from build123d import *

# Parameters (mm, degrees)
SKETCH1_R               = 6.5
BOSS_EXTRUDE1_DEPTH     = 4.64
SKETCH2_R               = 5.075
BOSS_EXTRUDE2_DEPTH     = 2
BOSS_EXTRUDE3_START     = 2
SKETCH3_R               = 5.075
BOSS_EXTRUDE3_DEPTH     = 2
SKETCH4_R               = 3.175
CUT_EXTRUDE1_DEPTH      = 13.615450844
CUT_EXTRUDE2_DEPTH      = 12.339735447
CUT_EXTRUDE2_DEPTH_BACK = 12.339735447
CUT_EXTRUDE3_DEPTH      = 12.339735447
CUT_EXTRUDE3_DEPTH_BACK = 12.339735447
SKETCH6_W               = 1
SKETCH6_H               = 2


with BuildPart() as part:
    # Sketch1 → Boss-Extrude1 (new body)
    with BuildSketch(Plane(origin=(0, 0, 0), x_dir=(1, 0, 0), z_dir=(0, 1, 0))):
        with Locations(Location((0, 0, 0), (0, 0, 270))):
            Circle(SKETCH1_R)
    extrude(amount=BOSS_EXTRUDE1_DEPTH)

    # Sketch2 → Boss-Extrude2 (add)
    with BuildSketch(Plane(origin=(0, 4.64, 0), x_dir=(1, 0, 0), z_dir=(0, 1, 0))):
        with Locations(Location((0, 0, 0), (0, 0, 270))):
            Circle(SKETCH2_R)
    extrude(amount=BOSS_EXTRUDE2_DEPTH)

    # Sketch3 → Boss-Extrude3 (add)
    with BuildSketch(Plane.XZ.offset(BOSS_EXTRUDE3_START)):
        with Locations(Location((0, 0, 0), (0, 0, 90))):
            Circle(SKETCH3_R)
    extrude(amount=-BOSS_EXTRUDE3_DEPTH)

    # Sketch4 → Cut-Extrude1 (cut, through all)
    with BuildSketch(Plane(origin=(0, 6.64, 0), x_dir=(1, 0, 0), z_dir=(0, 1, 0))):
        with Locations(Location((0, 0, 0), (0, 0, 270))):
            Circle(SKETCH4_R)
    extrude(amount=-CUT_EXTRUDE1_DEPTH, mode=Mode.SUBTRACT)

    # Sketch5 → Cut-Extrude2 (cut, two sides: drawn at the far end of the back side and taken through both)
    with BuildSketch(Plane.XY.offset(-CUT_EXTRUDE2_DEPTH_BACK)):
        Polygon((0, 0), (-1, 0), (-1, -2), (1, -2), (1, 0), align=None)
    extrude(amount=CUT_EXTRUDE2_DEPTH + CUT_EXTRUDE2_DEPTH_BACK, mode=Mode.SUBTRACT)

    # Sketch6 → Cut-Extrude3 (cut, two sides: drawn at the far end of the back side and taken through both)
    with BuildSketch(Plane(origin=(0, 0, 0), x_dir=(0, 0, -1), z_dir=(1, 0, 0)).offset(-CUT_EXTRUDE3_DEPTH_BACK)):
        with Locations((0.5, -1)):
            Rectangle(SKETCH6_W, SKETCH6_H)
        with Locations((-0.5, -1)):
            Rectangle(SKETCH6_W, SKETCH6_H)
    extrude(amount=CUT_EXTRUDE3_DEPTH + CUT_EXTRUDE3_DEPTH_BACK, mode=Mode.SUBTRACT)


solid = part.part
Input: part model. Units: mm. Frame: model coordinates. A direction names the side the tool comes from. Give positions to 0.01 mm unless a question says otherwise; leave off trailing zeros. Write each loop counter-clockwise with the first axis right and the second up, starting at its lowest first coordinate (ties: lowest second). Pieces come first, ordered by that corner, then holes.
Q1. Section C-C, the plane y = 5.25. Output: boundary loops of the cut face in (x, z) (3 decimals), plus the area to 3 significant figures.
Q2. Pull-direction query (Z, two-part tool) for faces 6 (the face through (-1, -1, 4)), 7 (the face through (3.559, -1.014, -3.618)), 8 (the face through (-4, -1, 1)); classes: pulls with the +Z half, pulls with the -Z half, needs draft (parallel to the pull), parting line crosses it, or undercut.
Q3. Material intervals for probe 1 along X at (y, z) = (4, 0) (3 decimals); probe 2 along X at (y, z) = (4.75, 0) (3 decimals); probe 3 along Y at (x, z) = (5, -2), sorted ascending.
Q4. Section D-D, the plane x = 3.75. Output: boundary loops of the cut face in (y, z).
Q5. Section A-A, the plane x = 0. Output: boundary loops of the cut face in (y, z) (3 decimals).
Q6. Section B-B, the plane z = 0. Output: boundary loops of the cut face in (x, y) (3 decimals), plus the area to 3 significant figures.
Q7. Set-up query: faces 1 (the face through (-5, 4.64, -2)), 2 (the face through (4, -1, -1)), 3 (the face through (3.618, -1.014, 3.559)), 4 (the face through (1, -1, -4)), 5 (the face through (-3.559, -1.014, 3.618)). Return all of +Z, -Z, +X, -X, +Y, -Y with unobstructed straight access to the full face (end or side cutting, diameter ignored); none if empty.
Q8. First-contact query: P1, Ø1.5, axis at x = 1.5, z = -5, coming from the -Y side; P2, Ø3, axis at y = 2, z = 3.5, coming from the +X side; P3, Ø1, axis at x = 4.5, y = -1, coming from the +Z side; P4, Ø4, axis at y = 5.5, z = -2, coming from the -X side. Flat tips, straight axial feed; report the tip coordinate or a pass-through.
Filled in:
1. outline: circle Ø10.15 at (0, 0); hole circle Ø6.35 at (0, 0)
1. area: 49.2 mm2
2. face 6: needs draft
2. face 7: pulls with the -Z half
2. face 8: undercut
3. probe 1: x = -6.5 to -3.175, 3.175 to 6.5
3. probe 2: x = -5.075 to -3.175, 3.175 to 5.075
3. probe 3: y = 0 to 4.64
4. outline: (-2, -3.42) - (0, -3.42) - (0, -5.31) - (4.64, -5.31) - (4.64, -3.42) - (6.64, -3.42) - (6.64, 3.42) - (4.64, 3.42) - (4.64, 5.31) - (0, 5.31) - (0, 3.42) - (-2, 3.42) - (-2, 1) - (0, 1) - (0, -1) - (-2, -1) - close
5. outline: (0, -6.5) - (4.64, -6.5) - (4.64, -5.075) - (6.64, -5.075) - (6.64, -3.175) - (0, -3.175) - close; (0, 3.175) - (6.64, 3.175) - (6.64, 5.075) - (4.64, 5.075) - (4.64, 6.5) - (0, 6.5) - close
6. outline: (-6.5, 0) - (-3.175, 0) - (-3.175, 6.64) - (-5.075, 6.64) - (-5.075, 4.64) - (-6.5, 4.64) - close; (3.175, 0) - (6.5, 0) - (6.5, 4.64) - (5.075, 4.64) - (5.075, 6.64) - (3.175, 6.64) - close
6. area: 38.5 mm2
7. face 1: +Y
7. face 2: +X, -X, -Y
7. face 3: +Z, +X, -Y
7. face 4: +Z, -Z, -Y
7. face 5: +Z, -X, -Y
8. P1: stops at y = -2
8. P2: stops at x = 6.18
8. P3: stops at z = 3.12
8. P4: stops at x = -6.5
